Design review of the part built by this model. Coordinates are the model's own, in mm. Give positions to 0.01 mm unless a question says otherwise; leave off trailing zeros. Write each loop counter-clockwise with the first axis right and the second up, starting at its lowest first coordinate (ties: lowest second). Pieces come first, ordered by that corner, then holes. Notation, with made-up numbers: (10, -38) -> (59, -38) arc R19 cw to (59, -6) -> close; hole circle Ø11 at (40, 70.25). An arc over 180 degrees is marked (long way). Answer as a JSON object with one key per item and string values.
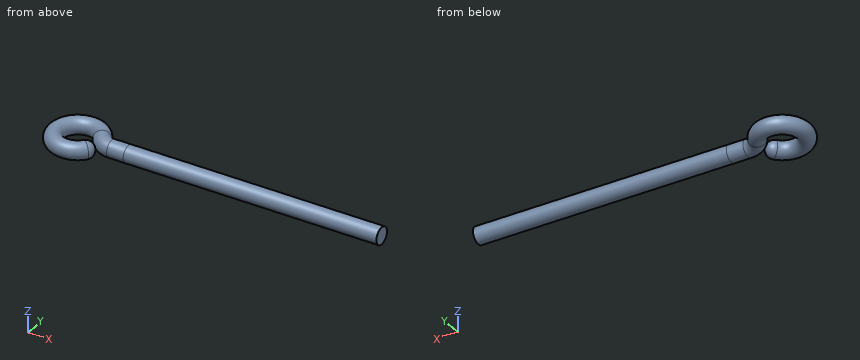
```python
from build123d import *

# Parameters (mm, degrees)
SKETCH2_R           = 5
DOME3_FACE_RADIUS   = 5
DOME3_HEIGHT        = 5
SKETCH4_R           = 5
BOSS_EXTRUDE2_DEPTH = 150


with BuildPart() as part:
    # Sweep2: sweep along a path in Sketch1
    with BuildLine(Plane.XY) as sweep2_path:
        Line((0, 0), (-9.844355629, 0))
        ThreePointArc((-9.844355629, 0), (-15.114818396, 1.501634144), (-18.802419794, 5.555555556))
        ThreePointArc((-18.802419794, 5.555555556), (-42.411911207, 1.481371052), (-20.424444461, -8.034845121))
    # Sketch2 → Sweep2 (sweep)
    with BuildSketch(Plane(origin=(0, 0, 0), x_dir=(0, 0, -1), z_dir=(1, 0, 0))):
        Circle(SKETCH2_R)
    sweep(path=sweep2_path.line)

    # Dome3: a dome of height H over a round flat face of radius A is a cap of a sphere of radius (A * A + H * H) / (2 * H)
    dome3_r = (DOME3_FACE_RADIUS * DOME3_FACE_RADIUS + DOME3_HEIGHT * DOME3_HEIGHT) / (2 * DOME3_HEIGHT)
    dome3_base = Plane((-20.424444461, -8.034845121, 0), z_dir=(0.64278761, 0.766044443, 0))
    with Locations(dome3_base.offset(DOME3_HEIGHT - dome3_r)):
        dome3_ball = Sphere(dome3_r, mode=Mode.PRIVATE)
    add(split(dome3_ball, bisect_by=dome3_base, keep=Keep.TOP, mode=Mode.PRIVATE))

    # Sketch4 → Boss-Extrude2 (add)
    with BuildSketch(Plane(origin=(0, 0, 0), x_dir=(0, 0, -1), z_dir=(1, 0, 0))):
        Circle(SKETCH4_R)
    extrude(amount=BOSS_EXTRUDE2_DEPTH)


solid = part.part
```
(1) For line 1 along Y through (x, z) = (-30, 2.5); line 2 along X through (y, z) = (1, -4); line 3 along Y through (x, z) = (75, -0.5), list the stretches that pass through material, from the lowest coordinate up.
Here are the results:
{"line 1": "y = -16.83 to -8.17, 8.17 to 16.83", "line 2": "x = -45.47 to -39.45, -19.23 to 150", "line 3": "y = -4.97 to 4.97"}
(2) Clearance check with flat-ended pins moving along their axes: pin 1 (5 mm diameter, centred on x = 117, y = -1, fed in from -Z); pin 2 (4 mm diameter, centred on x = 118.5, z = -4, fed in from -Y); pin 3 (4 mm diameter, centred on x = -24.5, y = -5, fed in from +Z). State where each tip first meets the part, or that it passes through.
Here are the results:
{"pin 1": "stops at z = -5", "pin 2": "stops at y = -4.58", "pin 3": "stops at z = 3.95"}
(3) We need section B-B, the plane x = 93. State the section outline as (y, z) points, then the cut area to 3 significant figures.
Here are the results:
{"outline": "circle Ø10 at (0, 0)", "area": "78.5 mm²"}
(4) We need section A-A, the plane z = 0. State the section outline as (x, y) points.
Here are the results:
{"outline": "(-24.25, -4.82) arc R7.5 cw (long way) to (-23.28, 3.33) arc R15 ccw to (-9.84, -5) -> (150, -5) -> (150, 5) -> (-9.84, 5) arc R5 cw to (-14.32, 7.78) arc R17.5 ccw (long way) to (-16.59, -11.25) arc R5 ccw to start"}
